```python
from build123d import *

# Parameters (mm, degrees)
F1_W     = 25.4
F1_H     = 3.175
F4_DEPTH = 76.2
F2_W     = 25.4
F2_H     = 3.175
F3_W     = 25.4
F3_H     = 3.175
F0_W     = 342.9
F0_H     = 12.7


with BuildPart() as f4:
    # F1 (on face) → F4 (new body, symmetric)
    with BuildSketch(Plane.XZ):
        with Locations((-247.65, 0)):
            Rectangle(F1_W, F1_H)
    extrude(amount=F4_DEPTH, both=True)



with BuildPart() as f4b:
    # F2 (on face) → F4, piece 2 (new body, symmetric)
    with BuildSketch(Plane.XZ):
        with Locations((-171.45, 0)):
            Rectangle(F2_W, F2_H)
    extrude(amount=F4_DEPTH, both=True)


with BuildPart() as f4c:
    # F3 (on face) → F4, piece 3 (new body, symmetric)
    with BuildSketch(Plane.XZ):
        with Locations((-95.25, 0)):
            Rectangle(F3_W, F3_H)
    extrude(amount=F4_DEPTH, both=True)


with BuildPart() as f4_1:
    add(f4.part)

    add(f4b.part)  # F5 merges F4b

    add(f4c.part)  # F5 merges F4c
    # F0 (on Front) → F5 (revolve)
    with BuildSketch(Plane.XZ):
        with Locations((-171.45, 6.35)):
            Rectangle(F0_W, F0_H)
    revolve(axis=Axis((-171.45, 0, 0), (-1, 0, 0)))


solid = f4_1.part
```
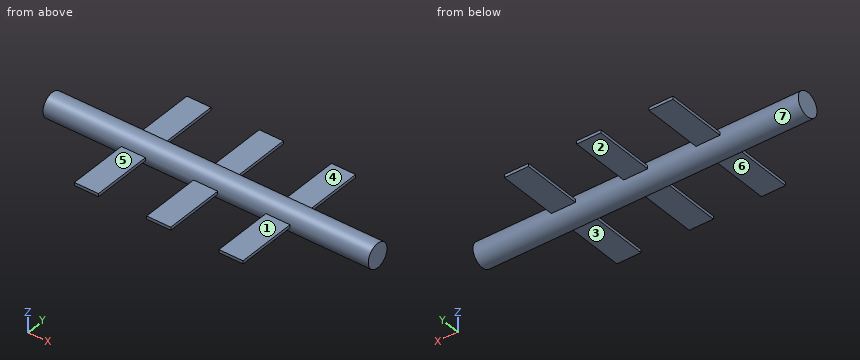
The model under review builds one solid part; all positions refer to its coordinate system, in mm. Face numbers are marked on the shaded views. A direction names the side the tool comes from. Coordinates: 2 decimals unless noted, no trailing zeros. Loops run counter-clockwise (first coordinate to the right, second up) from the corner with the lowest first, then second, coordinate; pieces in that order, holes last. Notation, with made-up numbers: (-36.75, 27) -> (-6.75, 27) arc R16 cw to (-6.75, 50) -> close; hole circle Ø7 at (0.5, 55.5). An arc over 180 degrees is marked (long way). Answer as CSV lines item,"result".
Item 1: Machinability: for the marked faces 1, 2, 3 and 4, which of the approach directions +Z, -Z, +X, -X, +Y, -Y give a long, thin tool a straight path to every point of the face, cutting with its end or side? Answer none if there is none.
Results below:
face 1,"+Z, +X, -X, -Y"
face 2,"-Z, +X, -X, +Y"
face 3,"-Z, +X, -X, -Y"
face 4,"+Z, +X, -X, +Y"
Item 2: Take a section at C-C, the plane z = -8. State the section outline as (x, y) points, and give its area (3 significant figures).
Results below:
outline,"(-342.9, -9.86) -> (0, -9.86) -> (0, 9.86) -> (-342.9, 9.86) -> close"
area,"6,760 mm2"
Item 3: For L1, parallel to X at y = -44, z = -1.25; L2, parallel to Z at x = -173, y = 53; L3, parallel to Y at x = -127, z = -1.5, list the stretches that pass through material, from the lowest coordinate up.
Results below:
L1,"x = -260.35 to -234.95, -184.15 to -158.75, -107.95 to -82.55"
L2,"z = -1.59 to 1.59"
L3,"y = -12.61 to 12.61"
Item 4: Draft analysis for pull direction Z (two halves, no side actions). For the marked faces 5, 6 and 7, state which applies: +Z half, -Z half, draft (parallel to the pull), parting line (faces both ways), or undercut.
Results below:
face 5,"+Z half"
face 6,"-Z half"
face 7,"parting line"
Item 5: Insertion check: pin 1 (20.5 mm diameter, centred on x = -252, y = -36, fed in from -Z); pin 2 (2.5 mm diameter, centred on y = -58.5, z = 0, fed in from -X); pin 3 (2.5 mm diameter, centred on y = 33.5, z = 0.5, fed in from +X); pin 4 (1.5 mm diameter, centred on y = -37.5, z = 3.5, fed in from +X). Each pin has a flat end and moves straight along its axis. Give the tip position at first contact, or say it passes through.
Results below:
pin 1,"stops at z = -1.59"
pin 2,"stops at x = -260.35"
pin 3,"stops at x = -82.55"
pin 4,"passes through"
Item 6: Take a section at B-B, the plane z = 6. State the section outline as (x, y) points.
Results below:
outline,"(-342.9, -11.19) -> (0, -11.19) -> (0, 11.19) -> (-342.9, 11.19) -> close"
Item 7: Take a section at A-A, the plane y = 37. State the section outline as (x, z) points, and give its area (3 significant figures).
Results below:
outline,"(-260.35, -1.59) -> (-234.95, -1.59) -> (-234.95, 1.59) -> (-260.35, 1.59) -> close; (-184.15, -1.59) -> (-158.75, -1.59) -> (-158.75, 1.59) -> (-184.15, 1.59) -> close; (-107.95, -1.59) -> (-82.55, -1.59) -> (-82.55, 1.59) -> (-107.95, 1.59) -> close"
area,"242 mm2"
